from build123d import *

# Parameters (mm, degrees)
SKETCH1_R                                      = 15
SKETCH1_R_2                                    = 5.5
BODY_DEPTH                                     = 4.7625
HEX_NUTYFOOT_DEPTH                             = 3.81
F_4_CLEARANCE_HOLE1_D                          = 3.2639
HEX_NUT_RECESS_DEPTH                           = 3.048
CSK_FOR_6_FLAT_HEAD_MACHINE_SCREW1_D           = 3.7973
CSK_FOR_6_FLAT_HEAD_MACHINE_SCREW1_CSINK_D     = 7.0866
CSK_FOR_6_FLAT_HEAD_MACHINE_SCREW1_CSINK_ANGLE = 82
FILLET1_R                                      = 2.54
FILLET2_R                                      = 1.27


with BuildPart() as part:
    # Sketch1 → Body (new body)
    # profile 1 of 5: a face of its own
    with BuildSketch(Plane.XY):
        Circle(SKETCH1_R)
        with Locations(Location((0, 0, 0), (0, 0, 180))):
            Circle(SKETCH1_R_2, mode=Mode.SUBTRACT)
    # profile 2 of 5: a face of its own
    with BuildSketch(Plane.XY):
        with BuildLine():
            ThreePointArc((-9, 12), (-4.74341649, 14.230249471), (0, 15))
            Line((0, 15), (0, 32.5))
            ThreePointArc((0, 32.5), (-4.544652323, 32.180679534), (-9, 31.228992939))
            Line((-9, 31.228992939), (-9, 12))
        make_face()
    # profile 3 of 5: a face of its own
    with BuildSketch(Plane.XY):
        with BuildLine():
            Line((0, 32.5), (0, 15))
            ThreePointArc((0, 15), (4.74341649, 14.230249471), (9, 12))
            Line((9, 12), (9, 31.228992939))
            ThreePointArc((9, 31.228992939), (4.544652323, 32.180679534), (0, 32.5))
        make_face()
    # profile 4 of 5: a face of its own
    with BuildSketch(Plane.XY):
        with BuildLine():
            ThreePointArc((-9, 31.228992939), (-4.544652323, 32.180679534), (0, 32.5))
            Line((0, 32.5), (0, 56))
            Line((0, 56), (-9, 56))
            Line((-9, 56), (-9, 31.228992939))
        make_face()
    # profile 5 of 5: a face of its own
    with BuildSketch(Plane.XY):
        with BuildLine():
            Line((0, 56), (0, 32.5))
            ThreePointArc((0, 32.5), (4.544652323, 32.180679534), (9, 31.228992939))
            Line((9, 31.228992939), (9, 56))
            Line((9, 56), (0, 56))
        make_face()
    extrude(amount=BODY_DEPTH)

    # Sketch1_3 → Hex NutyFoot (add)
    with BuildSketch(Plane.XY):
        with BuildLine():
            Line((0, 56), (0, 32.5))
            ThreePointArc((0, 32.5), (4.544652323, 32.180679534), (9, 31.228992939))
            Line((9, 31.228992939), (9, 56))
            Line((9, 56), (0, 56))
        make_face()
        with BuildLine():
            ThreePointArc((-9, 31.228992939), (-4.544652323, 32.180679534), (0, 32.5))
            Line((0, 32.5), (0, 56))
            Line((0, 56), (-9, 56))
            Line((-9, 56), (-9, 31.228992939))
        make_face()
    extrude(amount=-HEX_NUTYFOOT_DEPTH)

    # 4 Clearance Hole1 (through all)
    with Locations(Plane(origin=(0, 45.78, 4.7625), x_dir=(1, 0, 0), z_dir=(0, 0, 1))):
        with Locations((0, 0), (0, 6)):
            Hole(F_4_CLEARANCE_HOLE1_D / 2)

    # Sketch7 → Hex Nut Recess (cut)
    with BuildSketch(Plane(origin=(0, 0, -3.81), x_dir=(-1, 0, 0), z_dir=(0, 0, -1))):
        with BuildLine():
            ThreePointArc((0.815975, 53.193310158), (1.413310158, 52.595975), (1.63195, 51.78))
            Line((1.63195, 51.78), (2.667, 51.78))
            Line((2.667, 51.78), (1.3335, 54.089689752))
            Line((1.3335, 54.089689752), (0.815975, 53.193310158))
        make_face()
        with BuildLine():
            Line((2.667, 51.78), (1.63195, 51.78))
            ThreePointArc((1.63195, 51.78), (1.413310158, 50.964025), (0.815975, 50.366689842))
            Line((0.815975, 50.366689842), (1.3335, 49.470310248))
            Line((1.3335, 49.470310248), (2.667, 51.78))
        make_face()
        with BuildLine():
            Line((1.3335, 49.470310248), (0.815975, 50.366689842))
            ThreePointArc((0.815975, 50.366689842), (0, 50.14805), (-0.815975, 50.366689842))
            Line((-0.815975, 50.366689842), (-1.3335, 49.470310248))
            Line((-1.3335, 49.470310248), (1.3335, 49.470310248))
        make_face()
        with BuildLine():
            ThreePointArc((-0.815975, 50.366689842), (-1.413310158, 50.964025), (-1.63195, 51.78))
            Line((-1.63195, 51.78), (-2.667, 51.78))
            Line((-2.667, 51.78), (-1.3335, 49.470310248))
            Line((-1.3335, 49.470310248), (-0.815975, 50.366689842))
        make_face()
        with BuildLine():
            Line((-2.667, 51.78), (-1.63195, 51.78))
            ThreePointArc((-1.63195, 51.78), (-1.413310158, 52.595975), (-0.815975, 53.193310158))
            Line((-0.815975, 53.193310158), (-1.3335, 54.089689752))
            Line((-1.3335, 54.089689752), (-2.667, 51.78))
        make_face()
        with BuildLine():
            ThreePointArc((-0.815975, 53.193310158), (0, 53.41195), (0.815975, 53.193310158))
            Line((0.815975, 53.193310158), (1.3335, 54.089689752))
            Line((1.3335, 54.089689752), (-1.3335, 54.089689752))
            Line((-1.3335, 54.089689752), (-0.815975, 53.193310158))
        make_face()
        with BuildLine():
            ThreePointArc((0.815975, 47.193310158), (1.413310158, 46.595975), (1.63195, 45.78))
            Line((1.63195, 45.78), (2.667, 45.78))
            Line((2.667, 45.78), (1.3335, 48.089689752))
            Line((1.3335, 48.089689752), (0.815975, 47.193310158))
        make_face()
        with BuildLine():
            Line((2.667, 45.78), (1.63195, 45.78))
            ThreePointArc((1.63195, 45.78), (1.413310158, 44.964025), (0.815975, 44.366689842))
            Line((0.815975, 44.366689842), (1.3335, 43.470310248))
            Line((1.3335, 43.470310248), (2.667, 45.78))
        make_face()
        with BuildLine():
            Line((1.3335, 43.470310248), (0.815975, 44.366689842))
            ThreePointArc((0.815975, 44.366689842), (0, 44.14805), (-0.815975, 44.366689842))
            Line((-0.815975, 44.366689842), (-1.3335, 43.470310248))
            Line((-1.3335, 43.470310248), (1.3335, 43.470310248))
        make_face()
        with BuildLine():
            ThreePointArc((-0.815975, 44.366689842), (-1.413310158, 44.964025), (-1.63195, 45.78))
            Line((-1.63195, 45.78), (-2.667, 45.78))
            Line((-2.667, 45.78), (-1.3335, 43.470310248))
            Line((-1.3335, 43.470310248), (-0.815975, 44.366689842))
        make_face()
        with BuildLine():
            Line((-2.667, 45.78), (-1.63195, 45.78))
            ThreePointArc((-1.63195, 45.78), (-1.413310158, 46.595975), (-0.815975, 47.193310158))
            Line((-0.815975, 47.193310158), (-1.3335, 48.089689752))
            Line((-1.3335, 48.089689752), (-2.667, 45.78))
        make_face()
        with BuildLine():
            ThreePointArc((-0.815975, 47.193310158), (0, 47.41195), (0.815975, 47.193310158))
            Line((0.815975, 47.193310158), (1.3335, 48.089689752))
            Line((1.3335, 48.089689752), (-1.3335, 48.089689752))
            Line((-1.3335, 48.089689752), (-0.815975, 47.193310158))
        make_face()
    extrude(amount=-HEX_NUT_RECESS_DEPTH, mode=Mode.SUBTRACT)

    # CSK for _6 Flat Head Machine Screw1 (through all)
    with Locations(Plane(origin=(0, 10, 4.7625), x_dir=(1, 0, 0), z_dir=(0, 0, 1))):
        with Locations((0, 0), (8.660254038, -15), (-8.660254038, -15)):
            CounterSinkHole(CSK_FOR_6_FLAT_HEAD_MACHINE_SCREW1_D / 2, CSK_FOR_6_FLAT_HEAD_MACHINE_SCREW1_CSINK_D / 2, counter_sink_angle=CSK_FOR_6_FLAT_HEAD_MACHINE_SCREW1_CSINK_ANGLE)

    # Fillet1
    fillet1_edges = [part.edges().sort_by_distance(p)[0] for p in [
        (9, 56, 0.47625),
        (-9, 56, 0.47625),
    ]]
    fillet(fillet1_edges, radius=FILLET1_R)

    # Fillet2
    fillet2_edges = [part.edges().sort_by_distance(p)[0] for p in [
        (-9, 42.34449647, -3.81),
        (-8.256051224, 55.256051224, -3.81),
        (0, 56, -3.81),
        (8.256051224, 55.256051224, -3.81),
        (-9, 31.228992939, -1.905),
        (9, 31.228992939, -1.905),
        (0, 32.5, -3.81),
        (9, 42.34449647, -3.81),
    ]]
    fillet(fillet2_edges, radius=FILLET2_R)


solid = part.part
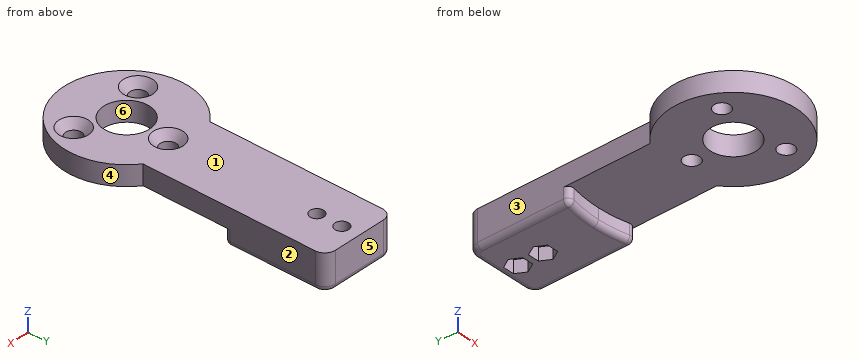
Part model, mm, in its own coordinate system. Face numbers are marked on the shaded views. A direction names the side the tool comes from. Coordinates: 2 decimals unless noted, no trailing zeros. Loops run counter-clockwise (first coordinate to the right, second up) from the corner with the lowest first, then second, coordinate; pieces in that order, holes last. Notation, with made-up numbers: M 21.5,-22 L 55.5,-22 A27 cw 55.5,7 Z; hole C -26.75,21 d5. An arc over 180 degrees is marked long. Use a Markdown table: item, result. Add a question column.
Q1. Cut at B-B (y = 10). Write the cut outline in (x, z), and give its area (3 significant figures).
Q2. Probe L1, parallel to Y at x = 0, z = 1.4; L2, parallel to X at y = 51.78, z = 2.1; L3, parallel to X at y = -5, z = 1.2. List the from-to ranges inside material, lowest first.
Q3. Mould opens along X. For the marked faces 4, 5 and 6 say: +X half, -X half, draft (parallel to the pull), parting line (faces both ways), or undercut.
Q4. Pin check, flat tips, straight feed: P1, Ø5, axis at x = -12, z = 2, coming from the +Y side; P2, Ø2.5, axis at x = 0, y = 10, coming from the +Z side; P3, Ø12, axis at x = 11.5, y = 3, coming from the -Z side; P4, Ø2, axis at y = 40, z = 2.5, coming from the -X side. Stop position of each tip, or through.
Q5. Which spindle directions (+Z, -Z, +X, -X, +Y, -Y) get a long thin tool onto all of the face, cutting with end or side? Do the marked faces 1, 2 and 3. Say none if no direction does.
Q6. Cut at C-C (y = 40.5). Write the cut outline in (x, z), and give its area (3 significant figures).
Q7. Cut at D-D (z = 4). Write the cut outline in (x, y).
Q8. Cut at A-A (z = 1.25). Write the cut outline in (x, y).
Worked out:
| question | item | result |
|---|---|---|
| 1 | outline | M -11.18,0 L -1.9,0 L -1.9,2.87 L -3.54,4.76 L -11.18,4.76 Z; M 1.9,0 L 11.18,0 L 11.18,4.76 L 3.54,4.76 L 1.9,2.87 Z |
| 1 | area | 85.3 mm2 |
| 2 | L1 | y = -15 to -5.5, 5.5 to 8.1, 11.9 to 44.15, 47.41 to 50.15, 53.41 to 56 |
| 2 | L2 | x = -9 to -1.63, 1.63 to 9 |
| 2 | L3 | x = -14.14 to -10.56, -6.76 to -2.29, 2.29 to 6.76, 10.56 to 14.14 |
| 3 | face 4 | parting line |
| 3 | face 5 | draft |
| 3 | face 6 | undercut |
| 4 | P1 | stops at y = 11.61 |
| 4 | P2 | passes through |
| 4 | P3 | stops at z = 0 |
| 4 | P4 | stops at x = -9 |
| 5 | face 1 | +Z, +X, -X, +Y, -Y |
| 5 | face 2 | +Z, -Z, +X, +Y |
| 5 | face 3 | +Z, -Z, -X, +Y |
| 6 | outline | M -9,-2.54 A1.27 ccw -7.73,-3.81 L 7.73,-3.81 A1.27 ccw 9,-2.54 L 9,4.76 L -9,4.76 Z |
| 6 | area | 154 mm2 |
| 7 | outline | M -9,12 A15 ccw long 9,12 L 9,53.46 A2.54 ccw 6.46,56 L -6.46,56 A2.54 ccw -9,53.46 Z; hole C -8.66,-5 d5.76; hole C 0,0 d11; hole C 0,10 d5.76; hole C 0,45.78 d3.26; hole C 0,51.78 d3.26; hole C 8.66,-5 d5.76 |
| 8 | outline | M -9,12 A15 ccw long 9,12 L 9,53.46 A2.54 ccw 6.46,56 L -6.46,56 A2.54 ccw -9,53.46 Z; hole C -8.66,-5 d3.8; hole C 0,0 d11; hole C 0,10 d3.8; hole C 0,45.78 d3.26; hole C 0,51.78 d3.26; hole C 8.66,-5 d3.8 |
